from build123d import *

# Parameters (mm, degrees)
EXTRUDE_1_DEPTH = 27.5
SKETCH_2_R      = 2.2
EXTRUDE_2_DEPTH = 3
SKETCH_3_W      = 40
SKETCH_3_H      = 20
EXTRUDE_3_DEPTH = 40
SKETCH_4_R      = 3
EXTRUDE_4_DEPTH = 7.5
FILLET_1_R      = 1


with BuildPart() as part:
    # ｽｹｯﾁ1 → ﾎﾞｽ - 押し出し1 (new body)
    with BuildSketch(Plane(origin=(0, 0, 0), x_dir=(0, 0, -1), z_dir=(1, 0, 0))):
        Polygon((40, 0), (0, 0), (0, -10), (0, -20), (40, -20), align=None)
    extrude(amount=EXTRUDE_1_DEPTH)

    # ｽｹｯﾁ2 → ﾎﾞｽ - 押し出し2 (add)
    with BuildSketch(Plane.ZY):
        with BuildLine():
            Line((5.5, 0), (-45.5, 0))
            ThreePointArc((-45.5, 0), (-46.914213562, -0.585786438), (-47.5, -2))
            Line((-47.5, -2), (-47.5, -18))
            ThreePointArc((-47.5, -18), (-46.914213562, -19.414213562), (-45.5, -20))
            Line((-45.5, -20), (5.5, -20))
            ThreePointArc((5.5, -20), (6.914213562, -19.414213562), (7.5, -18))
            Line((7.5, -18), (7.5, -2))
            ThreePointArc((7.5, -2), (6.914213562, -0.585786438), (5.5, 0))
        make_face()
        with Locations((-45, -5)):
            Circle(SKETCH_2_R, mode=Mode.SUBTRACT)
        with Locations(Location((5, -5, 0), (0, 0, 180))):
            Circle(SKETCH_2_R, mode=Mode.SUBTRACT)
        with Locations((5, -15)):
            Circle(SKETCH_2_R, mode=Mode.SUBTRACT)
        with Locations(Location((-45, -15, 0), (0, 0, 180))):
            Circle(SKETCH_2_R, mode=Mode.SUBTRACT)
    extrude(amount=EXTRUDE_2_DEPTH)

    # ｽｹｯﾁ3 → ﾎﾞｽ - 押し出し3 (add)
    with BuildSketch(Plane(origin=(27.5, 0, 0), x_dir=(0, 0, -1), z_dir=(1, 0, 0))):
        with Locations((20, -10)):
            Rectangle(SKETCH_3_W, SKETCH_3_H)
    extrude(amount=-EXTRUDE_3_DEPTH)

    # ｽｹｯﾁ4 → ﾎﾞｽ - 押し出し4 (add)
    with BuildSketch(Plane.ZY.offset(12.5)):
        with Locations(Location((-10, -10, 0), (0, 0, 180))):
            Circle(SKETCH_4_R)
    extrude(amount=EXTRUDE_4_DEPTH)

    # ﾌｨﾚｯﾄ1
    fillet_1_edges = [part.edges().sort_by_distance(p)[0] for p in [
        (27.5, 0, -20),
        (27.5, -10, 0),
        (27.5, -20, -20),
        (-7.75, -20, 0),
        (-7.75, 0, 0),
        (-7.75, 0, -40),
        (-7.75, -20, -40),
        (27.5, -10, -40),
        (13.75, -20, -40),
        (13.75, -20, 0),
        (13.75, 0, 0),
        (13.75, 0, -40),
    ]]
    fillet(fillet_1_edges, radius=FILLET_1_R)


solid = part.part
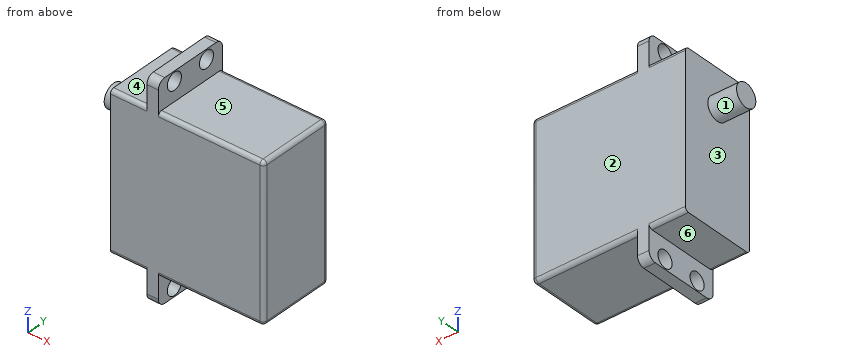
Verification items for the finished model (mm, model axes). Face numbers are marked on the shaded views. A direction names the side the tool comes from. Round coordinates to 2 decimals unless told otherwise and drop trailing zeros. Loops run counter-clockwise (first coordinate to the right, second up) from the corner with the lowest first, then second, coordinate; pieces in that order, holes last. Notation, with made-up numbers: (78.5, 10.5) - (128.5, 10.5) arc R18 ccw to (128.5, 25.5) - close; hole circle Ø6 at (67, -6). An arc over 180 degrees is marked (long way). Use a Markdown table: item, result. Add a question column.
1. Access from +Z, -Z, +X, -X, +Y, -Y to the whole of each face (thin tool, end or side, straight path). Record for the marked faces 4, 5 and 6.
2. Gauge pin test, flat ends, axial feed: pin 1 (4 mm diameter, centred on y = -12, z = 2.5, fed in from +X); pin 2 (1.5 mm diameter, centred on y = -2.5, z = -28, fed in from -X); pin 3 (9 mm diameter, centred on x = 17, y = -12, fed in from +Z). Record the tip position at first contact, or that the pin passes through.
3. Thickness scan on probe 1 along Y at (x, z) = (-0.75, 5); probe 2 along Z at (x, y) = (21, -5.5); probe 3 along X at (y, z) = (-6.5, -7.5). Record the ranges inside material, lowest first. Write a range as [from, to].
4. Section check A-A, the plane x = -4. Record the boundary of the cut face in (y, z).
5. Section check C-C, the plane z = -26. Record the boundary of the cut face in (x, y).
6. Release check for a two-part mould opening along Y. For the marked faces 1, 2 and 3 record: released by +Y, released by -Y, zero draft, split by the parting line, or undercut.
7. Section check D-D, the plane z = -10. Record the boundary of the cut face in (x, y).
8. Section check B-B, the plane y = -10. Record the boundary of the cut face in (x, z).
Checks:
| question | item | result |
|---|---|---|
| 1 | face 4 | +Z, -X, +Y, -Y |
| 1 | face 5 | +Z, +X, +Y, -Y |
| 1 | face 6 | -Z, -X, +Y, -Y |
| 2 | pin 1 | stops at x = 0 |
| 2 | pin 2 | stops at x = -12.5 |
| 2 | pin 3 | stops at z = 0 |
| 3 | probe 1 | y = [-20, -17.2], [-12.8, -7.2], [-2.8, 0] |
| 3 | probe 2 | z = [-40, 0] |
| 3 | probe 3 | x = [-12.5, 27.5] |
| 4 | outline | (-20, -39) arc R1 ccw to (-19, -40) - (-1, -40) arc R1 ccw to (0, -39) - (0, -1) arc R1 ccw to (-1, 0) - (-19, 0) arc R1 ccw to (-20, -1) - close |
| 5 | outline | (-12.5, -20) - (26.5, -20) arc R1 ccw to (27.5, -19) - (27.5, -1) arc R1 ccw to (26.5, 0) - (-12.5, 0) - close |
| 6 | face 1 | split by the parting line |
| 6 | face 2 | released by +Y |
| 6 | face 3 | zero draft |
| 7 | outline | (-20, -13) - (-12.5, -13) - (-12.5, -20) - (26.5, -20) arc R1 ccw to (27.5, -19) - (27.5, -1) arc R1 ccw to (26.5, 0) - (-12.5, 0) - (-12.5, -7) - (-20, -7) - close |
| 8 | outline | (-20, -13) - (-12.5, -13) - (-12.5, -40) - (-3, -40) - (-3, -47.5) - (0, -47.5) - (0, -40) - (26.5, -40) arc R1 ccw to (27.5, -39) - (27.5, -1) arc R1 ccw to (26.5, 0) - (0, 0) - (0, 7.5) - (-3, 7.5) - (-3, 0) - (-12.5, 0) - (-12.5, -7) - (-20, -7) - close |
